Check sheet for the modelled part. Datum: model origin and axes. Units: mm. A direction names the side the tool comes from. Give positions to 0.01 mm unless a question says otherwise; leave off trailing zeros. Loops run counter-clockwise (first coordinate to the right, second up) from the corner with the lowest first, then second, coordinate; pieces in that order, holes last.
```python
from build123d import *

# Parameters (mm, degrees)
F1_DEPTH      = 7.62
F0_W          = 3.81
F0_H          = 40.64
F2_DEPTH      = 17.78
F2_DEPTH_BACK = 7.62
F4_DEPTH      = 30.48
F6_DEPTH      = 50.8


# Not quite as in the source:
# - a feature names something its author has since deleted; it is built from what else it names


with BuildPart() as f1:
    # F0 (on Front) → F1 (new body)
    with BuildSketch(Plane.XZ):
        Polygon((-25.2661056346, 42.3477623217), (-55.7461056346, 42.3477623217), (-55.7461056346, 24.5677623217), (-51.9361056346, 24.5677623217), (-51.9361056346, -16.0722376783), (-55.7461056346, -16.0722376783), (-55.7461056346, -33.8522376783), (-25.2661056346, -33.8522376783), (-25.2661056346, -16.0722376783), (-29.0761056346, -16.0722376783), (-29.0761056346, 24.5677623217), (-25.2661056346, 24.5677623217), align=None)
    extrude(amount=F1_DEPTH)

    # F0 (on Front) → F2 (join, two sides)
    with BuildSketch(Plane.XZ) as f2_sk:
        with Locations((-53.8411056346, 4.2477623217)):
            Rectangle(F0_W, F0_H)
        with Locations((-27.1711056346, 4.2477623217)):
            Rectangle(F0_W, F0_H)
    extrude(amount=-F2_DEPTH)
    extrude(f2_sk.sketch, amount=F2_DEPTH_BACK)

    # F3 (on face) → F4 (join)
    with BuildSketch(Plane.YZ.offset(-25.2661056346)):
        with BuildLine():
            Line((-7.62, 42.3477623217), (0, 42.3477623217))
            Line((0, 42.3477623217), (0, 67.7477623217))
            Line((0, 67.7477623217), (-20.32, 67.7477623217))
            Line((-20.32, 67.7477623217), (-38.1, 49.9677623217))
            ThreePointArc((-38.1, 49.9677623217), (-30.341501455, -5.7914240632), (-12.7, -59.2522376783))
            Line((-12.7, -59.2522376783), (0, -59.2522376783))
            Line((0, -59.2522376783), (0, -33.8522376783))
            Line((0, -33.8522376783), (-7.62, -33.8522376783))
            Line((-7.62, -33.8522376783), (-7.62, 42.3477623217))
        make_face()
    extrude(amount=-F4_DEPTH)

    # F5 (on face) → F6 (cut)
    with BuildSketch(Plane.YZ.offset(-25.2661056346)):
        Polygon((0, 65.2077623217), (0, 67.7477623217), (-20.32, 67.7477623217), (-22.86, 65.2077623217), align=None)
    extrude(amount=-F6_DEPTH, mode=Mode.SUBTRACT)


solid = f1.part
```
(1) Section check A-A on y = 13.5. Record the boundary of the cut face in (x, z), plus the area to 3 significant figures.
(2) Material ranges on line 1 (Y direction, x = -40, z = 24); line 2 (Y direction, x = -34, z = -9.5), recorded low to high.
(3) Access from +Z, -Z, +X, -X, +Y, -Y to the whole of each face (thin tool, end or side, straight path). Record for faces 4 (the face through (-29.076, 9, 4)), 5 (the face through (-54, 9, -16.072)), 6 (the face through (-54, 9, 24.568)), 7 (the face through (-40.29, -30.52, -5.02)), 8 (the face through (-27, 17.78, 5)).
(4) Gauge pin test, flat ends, axial feed: pin 1 Ø3 at (x, y) = (-54, 5) entering from +Z; pin 2 Ø3 at (x, y) = (-54.5, 5.5) entering from -Z; pin 3 Ø1 at (x, y) = (-37, -13.5) entering from -Z. Record the tip position at first contact, or that the pin passes through.
(5) Section check D-D on y = -15. Record the boundary of the cut face in (x, z), plus the area to 3 significant figures.
(6) Section check B-B on x = -32.5. Record the boundary of the cut face in (y, z), plus the area to 3 significant figures.
(7) Release check for a two-part mould opening along X. For faces 1 (the face through (-40.293, -30.373, 57.694)), 2 (the face through (-55.746, -11, 4)), 3 (the face through (-51.936, 9, 4)) record: pulls with the +X half, pulls with the -X half, needs draft (parallel to the pull), parting line crosses it, or undercut.
(8) Section check C-C on z = 8.5. Record the boundary of the cut face in (x, y).
Computed values:
1. outline: (-55.75, -16.07) - (-51.94, -16.07) - (-51.94, 24.57) - (-55.75, 24.57) - close; (-29.08, -16.07) - (-25.27, -16.07) - (-25.27, 24.57) - (-29.08, 24.57) - close
1. area: 310 mm2
2. line 1: y = -35.76 to 0
2. line 2: y = -29.46 to 0
3. face 4: +Z, -Z, +Y
3. face 5: -Z, +X, -X, +Y
3. face 6: +Z, +X, -X, +Y
3. face 7: -Z, +X, -X, -Y
3. face 8: +Z, -Z, +X, -X, +Y
4. pin 1: stops at z = 24.57
4. pin 2: stops at z = -16.07
4. pin 3: stops at z = -58.56
5. outline: (-55.75, -53.8) - (-25.27, -53.8) - (-25.27, 65.21) - (-55.75, 65.21) - close
5. area: 3,630 mm2
6. outline: (-38.1, 49.97) arc R312.34 ccw to (-12.7, -59.25) - (0, -59.25) - (0, 65.21) - (-22.86, 65.21) - close
6. area: 3,620 mm2
7. face 1: needs draft
7. face 2: pulls with the -X half
7. face 3: undercut
8. outline: (-55.75, -33.31) - (-25.27, -33.31) - (-25.27, 17.78) - (-29.08, 17.78) - (-29.08, 0) - (-51.94, 0) - (-51.94, 17.78) - (-55.75, 17.78) - close
